Source: CAD feature listing. Evaluate the final solid. Frame: model axes, mm. Face numbers are marked on the shaded views. Give positions to 0.01 mm unless a question says otherwise; leave off trailing zeros. Loops run counter-clockwise (first coordinate to the right, second up) from the corner with the lowest first, then second, coordinate; pieces in that order, holes last. Notation, with made-up numbers: M 44.5,-2.75 L 69.5,-2.75 A15 cw 69.5,1.25 Z; hole C -2.75,-22.5 d5. An arc over 180 degrees is marked long. Answer in a Markdown table with one row per item.
```python
from build123d import *
from build123d.topology import SkipClean

# Parameters (mm, degrees)
BOSS_EXTRUDE1_DEPTH     = 74
CHAMFER1_SIZE           = 1
FILLET1_R               = 3
CUT_EXTRUDE1_DEPTH      = 121.138628729
CUT_EXTRUDE1_DEPTH_BACK = 121.138628729
CUT_EXTRUDE2_REACH      = 111.646
SKETCH4_R               = 1


with BuildPart() as part:
    # Sketch1 → Boss-Extrude1 (new, symmetric)
    with BuildSketch(Plane.XY):
        with BuildLine():
            Line((55.830466766, 51.361253738), (63.438083445, 57.851567172))
            ThreePointArc((63.438083445, 57.851567172), (72.243195979, 42.88470747), (75.398327752, 25.808934001))
            Line((75.398327752, 25.808934001), (65.398662212, 25.727147202))
            ThreePointArc((65.398662212, 25.727147202), (64.324262485, 34.614216947), (61.300381376, 43.039802177))
            Line((61.300381376, 43.039802177), (31.399799374, 25.449072083))
            Line((31.399799374, 25.449072083), (26.399966604, 25.408178684))
            ThreePointArc((26.399966604, 25.408178684), (25.395910676, 26.399991642), (24.40000005, 25.400000004))
            ThreePointArc((24.40000005, 25.400000004), (24.411675325, 25.24763781), (24.446428526, 25.098833357))
            Line((24.446428526, 25.098833357), (18.248213622, 23.141250154))
            ThreePointArc((18.248213622, 23.141250154), (17.987564613, 24.25728355), (17.90000005, 25.400000004))
            ThreePointArc((17.90000005, 25.400000004), (21.992343112, 32.081158151), (29.803433168, 31.471225314))
            Line((29.803433168, 31.471225314), (58.257984046, 48.211244769))
            ThreePointArc((58.257984046, 48.211244769), (57.083396924, 49.816436323), (55.830466766, 51.361253738))
        make_face()
    boss_extrude1 = extrude(amount=BOSS_EXTRUDE1_DEPTH, both=True)

    # Mirror1: Boss-Extrude1 across plane
    with SkipClean():  # the faces are left unmerged after this step: merging them gives an invalid solid
        add(boss_extrude1.mirror(Plane(origin=(-0.206032496, 25.190569454, 0), x_dir=(0, 0, 1), z_dir=(0.008178679945042752, -0.9999665540378622, 0))))

    # Chamfer1
    # the kernel refuses this chamfer: 1 mm, written as the material it takes off along each edge
    with BuildSketch(Plane(origin=(55.830466766, 51.361253738, -76.604800739), x_dir=(0.7607616678932755, 0.6490313433604278, 0), z_dir=(0, 0, 1))) as chamfer1_piece_1:
        with BuildLine():
            Line((CHAMFER1_SIZE, 0), (-0.01282473, -1.01282473))
            ThreePointArc((-0.01282473, -1.01282473), (-0.003390265, -0.520777989), (0, 0))
            Line((0, 0), (CHAMFER1_SIZE, 0))
        make_face()
    extrude(amount=153.209601479, mode=Mode.SUBTRACT)
    with BuildSketch(Plane(origin=(63.438083445, 57.851567172, 76.571682988), x_dir=(-0.7607616678932776, -0.6490313433604255, 0), z_dir=(0, 0, -1))) as chamfer1_piece_2:
        with BuildLine():
            Line((CHAMFER1_SIZE, 0), (0.009805807, -0.990194193))
            ThreePointArc((0.009805807, -0.990194193), (0.002592086, -0.509118755), (0, 0))
            Line((0, 0), (CHAMFER1_SIZE, 0))
        make_face()
    extrude(amount=153.143365976, mode=Mode.SUBTRACT)
    with BuildSketch(Plane(origin=(63.963798858, -6.425043932, 76.571682988), x_dir=(0.6288321665267481, 0.7775410640868277, 0), z_dir=(0, 0, -1))) as chamfer1_piece_3:
        with BuildLine():
            Line((0.990242745, 0), (CHAMFER1_SIZE * 0.00990242744899, -CHAMFER1_SIZE * 0.999950969763))
            Line((CHAMFER1_SIZE * 0.00990242744899, -CHAMFER1_SIZE * 0.999950969763), (0, 0))
            ThreePointArc((0, 0), (0.509119461, 0.002449552), (0.990242745, 0))
        make_face()
    extrude(amount=153.143365976, mode=Mode.SUBTRACT)
    with BuildSketch(Plane(origin=(56.251039097, -0.060035145, -76.604800739), x_dir=(0.6266844831673307, 0.7792730962616993, 0), z_dir=(0, 0, 1))) as chamfer1_piece_4:
        with BuildLine():
            Line((1.012905922, 0), (-CHAMFER1_SIZE * 0.0126613240298, -CHAMFER1_SIZE * 0.999919842224))
            Line((-CHAMFER1_SIZE * 0.0126613240298, -CHAMFER1_SIZE * 0.999919842224), (0, 0))
            ThreePointArc((0, 0), (0.520779169, -0.003203746), (1.012905922, 0))
        make_face()
    extrude(amount=153.209601479, mode=Mode.SUBTRACT)

    # Fillet1
    # the kernel refuses this fillet: 3 mm, written as the material it adds along each edge
    with BuildSketch(Plane(origin=(61.300381376, 43.039802177, 74), x_dir=(-0.8619070987590498, -0.5070662216207636, 0), z_dir=(0, 0, -1))) as fillet1_piece_1:
        with BuildLine():
            CenterArc((3.377068823, -3), FILLET1_R, 90, 99.332418184)
            Line((0.416776456, -3.486486486), (0.357570609, -3.496216216))
            ThreePointArc((0.357570609, -3.496216216), (0.110537283, -1.754940397), (-0.059831012, -0.0045))
            Line((-0.059831012, -0.0045), (0, 0.06))
            Line((0, 0.06), (3.377068823, 0.06))
            Line((3.377068823, 0.06), (3.377068823, 0))
        make_face()
    extrude(amount=148)
    with BuildSketch(Plane(origin=(31.399799374, 25.449072083, 74), x_dir=(0.861907098759051, 0.5070662216207618, 0), z_dir=(0, 0, -1))) as fillet1_piece_2:
        with BuildLine():
            CenterArc((FILLET1_R * 1.73205080757, FILLET1_R), FILLET1_R, 150, 120)
            Line((FILLET1_R * 0.866025403784, FILLET1_R * 1.5), (FILLET1_R * 0.848704895709, FILLET1_R * 1.51))
            Line((FILLET1_R * 0.848704895709, FILLET1_R * 1.51), (-FILLET1_R * 0.0346410161514, -FILLET1_R * 0.02))
            Line((-FILLET1_R * 0.0346410161514, -FILLET1_R * 0.02), (FILLET1_R * 1.73205080757, -FILLET1_R * 0.02))
            Line((FILLET1_R * 1.73205080757, -FILLET1_R * 0.02), (FILLET1_R * 1.73205080757, 0))
        make_face()
    extrude(amount=148)
    with BuildSketch(Plane(origin=(29.803433168, 31.471225314, -74), x_dir=(-0.8632427379298097, 0.5047890405025113, 0), z_dir=(0, 0, 1))) as fillet1_piece_3:
        with BuildLine():
            CenterArc((1.767704789, -2.985498375), FILLET1_R, 95.63586305, 55.150095421)
            Line((-0.850702684, -1.521277659), (-0.903070833, -1.491993244))
            Line((-0.903070833, -1.491993244), (-0.052368149, 0.029284414))
            Line((-0.052368149, 0.029284414), (0.005892349, 0.059709968))
            ThreePointArc((0.005892349, 0.059709968), (0.736543662, 0.023745938), (1.467194975, 0.059709968))
            Line((1.467194975, 0.059709968), (1.473087324, 0))
        make_face()
    extrude(amount=148)
    with BuildSketch(Plane(origin=(58.257984046, 48.211244769, -74), x_dir=(-0.6003331349359272, 0.7997500403863709, 0), z_dir=(0, 0, 1))) as fillet1_piece_4:
        with BuildLine():
            CenterArc((3.35394685, 2.974664865), FILLET1_R, 173.574848661, 88.973633867)
            Line((0.372790176, 3.310380343), (0.313167042, 3.317094653))
            Line((0.313167042, 3.317094653), (-0.059623133, 0.00671431))
            Line((-0.059623133, 0.00671431), (-0.002223664, -0.05995878))
            ThreePointArc((-0.002223664, -0.05995878), (1.482442617, -0.087479891), (2.957104003, -0.059493297))
            Line((2.957104003, -0.059493297), (2.964885235, 0))
        make_face()
    extrude(amount=148)
    with BuildSketch(Plane(origin=(61.584109507, 8.349773529, 74), x_dir=(-0.8700857787040926, 0.49290033241710485, 0), z_dir=(0, 0, -1))) as fillet1_piece_5:
        with BuildLine():
            CenterArc((3.377068823, 3), FILLET1_R, 170.667581816, 99.332418184)
            Line((0.416776456, 3.486486486), (0.357570609, 3.496216216))
            ThreePointArc((0.357570609, 3.496216216), (0.110537283, 1.754940397), (-0.059831012, 0.0045))
            Line((-0.059831012, 0.0045), (0, -0.06))
            Line((0, -0.06), (3.377068823, -0.06))
            Line((3.377068823, -0.06), (3.377068823, 0))
        make_face()
    extrude(amount=148)
    with BuildSketch(Plane(origin=(58.626707512, 3.129258857, -74), x_dir=(-0.870085778704093, 0.49290033241710457, 0), z_dir=(0, 0, 1))) as fillet1_piece_6:
        with BuildLine():
            CenterArc((3.331304629, 3), FILLET1_R, 181.026366133, 88.973633867)
            Line((0.331785955, 2.946262469), (0.271795581, 2.945187718))
            ThreePointArc((0.271795581, 2.945187718), (0.078962557, 1.482920686), (-0.059831012, 0.0045))
            Line((-0.059831012, 0.0045), (0, -0.06))
            Line((0, -0.06), (3.331304629, -0.06))
            Line((3.331304629, -0.06), (3.331304629, 0))
        make_face()
    extrude(amount=148)
    with BuildSketch(Plane(origin=(29.902149966, 19.401613043, -74), x_dir=(-0.8548705120852164, -0.5188414088786282, 0), z_dir=(0, 0, 1))) as fillet1_piece_7:
        with BuildLine():
            CenterArc((1.767704789, 2.985498375), FILLET1_R, 209.214041529, 55.150095421)
            Line((-0.850702684, 1.521277659), (-0.903070833, 1.491993244))
            Line((-0.903070833, 1.491993244), (-0.052368149, -0.029284414))
            Line((-0.052368149, -0.029284414), (0.005892349, -0.059709968))
            ThreePointArc((0.005892349, -0.059709968), (0.736543662, -0.023745938), (1.467194975, -0.059709968))
            Line((1.467194975, -0.059709968), (1.473087324, 0))
        make_face()
    extrude(amount=148)

    # Sketch3 → Cut-Extrude1 (cut, two sides: drawn at the far end of the back side and taken through both)
    with BuildSketch(Plane.XY.offset(-CUT_EXTRUDE1_DEPTH_BACK)):
        with BuildLine():
            Line((22.960409716, 23.368000004), (22.960409716, 27.432000004))
            ThreePointArc((22.960409716, 27.432000004), (28.57500005, 25.400000004), (22.960409716, 23.368000004))
        make_face()
        with BuildLine():
            Line((18.180514196, 27.432000004), (18.180514196, 23.368000004))
            ThreePointArc((18.180514196, 23.368000004), (17.90000005, 25.400000004), (18.180514196, 27.432000004))
        make_face()
    extrude(amount=CUT_EXTRUDE1_DEPTH + CUT_EXTRUDE1_DEPTH_BACK, mode=Mode.SUBTRACT)

    # Sketch4 → Cut-Extrude2 (cut, up to next)
    with BuildSketch(Plane.ZY.offset(-18.180514196), mode=Mode.PRIVATE) as cut_extrude2_sk1:
        with Locations((0, 25.400000004)):
            Circle(SKETCH4_R)
    cut_extrude2_tool1 = extrude(cut_extrude2_sk1.sketch, amount=-CUT_EXTRUDE2_REACH, mode=Mode.PRIVATE) & part.part
    # Sketch4 → Cut-Extrude2 (cut, up to next)
    with BuildSketch(Plane.ZY.offset(-18.180514196), mode=Mode.PRIVATE) as cut_extrude2_sk2:
        with Locations((30, 25.400000004)):
            Circle(SKETCH4_R)
    cut_extrude2_tool2 = extrude(cut_extrude2_sk2.sketch, amount=-CUT_EXTRUDE2_REACH, mode=Mode.PRIVATE) & part.part
    # Sketch4 → Cut-Extrude2 (cut, up to next)
    with BuildSketch(Plane.ZY.offset(-18.180514196), mode=Mode.PRIVATE) as cut_extrude2_sk3:
        with Locations((60, 25.400000004)):
            Circle(SKETCH4_R)
    cut_extrude2_tool3 = extrude(cut_extrude2_sk3.sketch, amount=-CUT_EXTRUDE2_REACH, mode=Mode.PRIVATE) & part.part
    # Sketch4 → Cut-Extrude2 (cut, up to next)
    with BuildSketch(Plane.ZY.offset(-18.180514196), mode=Mode.PRIVATE) as cut_extrude2_sk4:
        with Locations((-30, 25.400000004)):
            Circle(SKETCH4_R)
    cut_extrude2_tool4 = extrude(cut_extrude2_sk4.sketch, amount=-CUT_EXTRUDE2_REACH, mode=Mode.PRIVATE) & part.part
    # Sketch4 → Cut-Extrude2 (cut, up to next)
    with BuildSketch(Plane.ZY.offset(-18.180514196), mode=Mode.PRIVATE) as cut_extrude2_sk5:
        with Locations((-60, 25.400000004)):
            Circle(SKETCH4_R)
    cut_extrude2_tool5 = extrude(cut_extrude2_sk5.sketch, amount=-CUT_EXTRUDE2_REACH, mode=Mode.PRIVATE) & part.part
    add(cut_extrude2_tool1.solids().sort_by_distance((18.180514, 25.4, 0))[0], mode=Mode.SUBTRACT)
    add(cut_extrude2_tool2.solids().sort_by_distance((18.180514, 25.4, 30))[0], mode=Mode.SUBTRACT)
    add(cut_extrude2_tool3.solids().sort_by_distance((18.180514, 25.4, 60))[0], mode=Mode.SUBTRACT)
    add(cut_extrude2_tool4.solids().sort_by_distance((18.180514, 25.4, -30))[0], mode=Mode.SUBTRACT)
    add(cut_extrude2_tool5.solids().sort_by_distance((18.180514, 25.4, -60))[0], mode=Mode.SUBTRACT)


solid = part.part
```
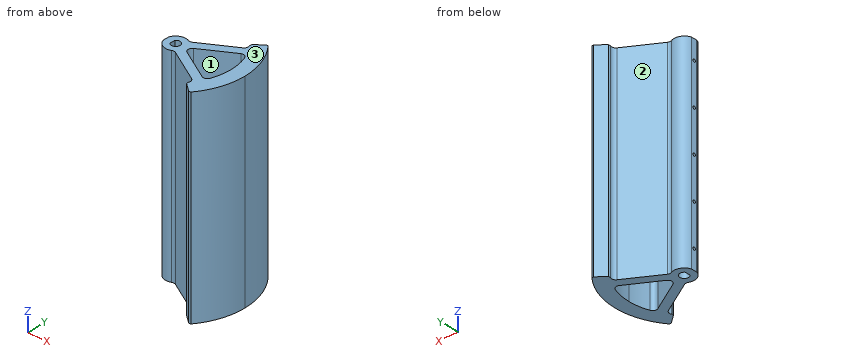
1) Pull-direction query (Y, two-part tool) for the marked faces 1, 2 and 3; classes: released by +Y, released by -Y, zero draft, split by the parting line, or undercut.
Reply:
| item | result |
|---|---|
| face 1 | undercut |
| face 2 | released by +Y |
| face 3 | zero draft |
2) Section C-C, the plane z = 16. Count the separate pieces of the cut face and the enclosed holes in it, then the cut area to 3 significant figures.
Reply:
| item | result |
|---|---|
| separate pieces | 1 |
| enclosed holes | 2 |
| area | 1,180 mm² |
3) Section B-B, the plane y = 37.5. Return loops of the section in (x, z).
Reply:
| item | result |
|---|---|
| outline | M 40.05,-74 L 51.88,-74 L 51.88,74 L 40.05,74 Z; M 63.53,-74 L 73.91,-74 L 73.91,74 L 63.53,74 Z |
4) Section A-A, the plane x = 25.4. Return loops of the section in (y, z) (3 decimals).
Reply:
| item | result |
|---|---|
| outline | M 17.9,-74 L 22.225,-74 L 22.225,74 L 17.9,74 Z; M 28.575,-74 L 32.9,-74 L 32.9,74 L 28.575,74 Z |
5) Material intervals for L1, parallel to X at y = 27.5, z = -5.5; L2, parallel to Z at x = 21, y = 25; L3, parallel to Y at x = 51.5, z = 36.5, sorted ascending.
Reply:
| item | result |
|---|---|
| L1 | x = 18.2 to 23.02, 27.78 to 35.17, 65.34 to 75.36 |
| L2 | z = -74 to -60.92, -59.08 to -30.92, -29.08 to -0.92, 0.92 to 29.08, 30.92 to 59.08, 60.92 to 74 |
| L3 | y = 7.17 to 14.06, 37.27 to 44.24 |
6) Pin query (flat end, axial travel): pin 1 Ø1 at (y, z) = (18.5, -47.5) entering from -X; pin 2 Ø12 at (y, z) = (36, 53) entering from -X; pin 3 Ø10 at (y, z) = (18.5, 18) entering from +X. Return the tip coordinate at first contact, or that it passes through.
Reply:
| item | result |
|---|---|
| pin 1 | stops at x = 21.49 |
| pin 2 | stops at x = 19.48 |
| pin 3 | stops at x = 75.36 |
